Autodesk Inventor part; units mm, degrees
ref_plane "YZ Plane" through (0, 0, 0) normal (1, 0, 0) x (0, 1, 0)
ref_plane "XZ Plane" through (0, 0, 0) normal (0, 1, 0) x (-1, 0, 0)
ref_plane "XY Plane" through (0, 0, 0) normal (0, 0, 1) x (1, 0, 0)
sketch "Sketch1" plane through (0, 0, 0) normal (0, 0, 1) x (1, 0, 0)
  line L0 (145, 65) -> (-145, 65)
  line L1 (-145, 65) -> (-145, -65)
  line L2 (-145, -65) -> (145, -65)
  line L3 (145, -65) -> (145, 65)
  line L4 (145, 65) -> (-145, -65) construction
  line L5 (-145, 65) -> (145, -65) construction
  line L6 (85, 40) -> (-115, 40)
  line L7 (-115, 40) -> (-115, -40)
  line L8 (-115, -40) -> (85, -40)
  line L9 (85, -40) -> (85, 40)
  line L10 (85, 40) -> (-115, -40) construction
  line L11 (-115, 40) -> (85, -40) construction
  point P0 (0, 0)
  point P1 (0, 0)
  point P2 (-15, 0)
  point P3 (85, 0)
  point P4 (145, 0)
  dimension "d34" = 200
  dimension "d35" = 80
  dimension "d51" = 60
  dimension "d53" = 30
  dimension "d54" = 25
  dimension "d56" = 130
extrude "Plate1" add sketch "Sketch1" along normal blind 2
sketch "Sketch6" plane through (145, -63.5858, 1.4142) normal (0, -0.7071068, -0.7071068) x (1, 0, 0)
  line L0 (-290, 0) -> (0, 0)
  line L1 (0, 0) -> (0, 70)
  line L2 (0, 70) -> (-290, 70)
  line L3 (-290, 70) -> (-290, 0)
edge flange "Flange2" height 70 angle 45 thickness 2 bend radius 2.75 thickness toward (0, -0.7071068, -0.7071068) relief round relief width 2 relief depth 1 edges at (0, -65, 2) wall of the first edge with corners at (-145, -63.5858, 1.4142) (145, -63.5858, 1.4142) (145, -113.0833, 50.9117) (-145, -113.0833, 50.9117)
bend "Bend2"
corner "Corner2"
sketch "Sketch8" plane through (145, -112.4975, 49.4975) normal (0, -1, 0) x (1, 0, 0)
  line L0 (-290, 0) -> (0, 0)
  line L1 (0, 0) -> (0, 130)
  line L2 (0, 130) -> (-290, 130)
  line L3 (-290, 130) -> (-290, 0)
edge flange "Flange3" height 130 angle 45 thickness 2 bend radius 2.75 thickness toward (0, -1, 0) relief round relief width 2 relief depth 1 edges at (0, -113.0833, 50.9117) wall of the first edge with corners at (-145, -112.4975, 49.4975) (145, -112.4975, 49.4975) (145, -112.4975, 179.4975) (-145, -112.4975, 179.4975)
bend "Bend3"
corner "Corner3"
sketch "Sketch9" plane through (145, -113.0833, 178.0833) normal (0, -0.7071068, 0.7071068) x (1, 0, 0)
  line L0 (-290, 0) -> (0, 0)
  line L1 (0, 0) -> (0, 68.6)
  line L2 (0, 68.6) -> (-290, 68.6)
  line L3 (-290, 68.6) -> (-290, 0)
edge flange "Flange4" height 68.6 angle 45 thickness 2 bend radius 2.75 thickness toward (0, -0.7071068, 0.7071068) relief round relief width 2 relief depth 1 edges at (0, -112.4975, 179.4975) wall of the first edge with corners at (-145, -113.0833, 178.0833) (145, -113.0833, 178.0833) (145, -64.5757, 226.5908) (-145, -64.5757, 226.5908)
bend "Bend4"
corner "Corner4"
sketch "Sketch10" plane through (-145, -114.4975, 51.465) normal (0, -1, 0) x (1, 0, 0)
  line L0 (290, 126.065) -> (0, 126.065)
  line L1 (0, 0) -> (0, 126.065)
  line L2 (0, 0) -> (290, 0)
  line L3 (290, 126.065) -> (290, 0)
  line L4 (30, 23.0325) -> (230, 23.0325)
  line L5 (230, 23.0325) -> (230, 103.0325)
  line L6 (230, 103.0325) -> (30, 103.0325)
  line L7 (30, 103.0325) -> (30, 23.0325)
  point P0 (145, -51.465)
  point P1 (30, 63.0325)
  point P2 (0, 63.0325)
  dimension "d77" = 80
  dimension "d78" = 200
  dimension "d79" = 30
extrude "Cut3" cut sketch "Sketch10" against normal blind 2 contours L7 L6 L5 L4
equation "\"d34\" = MAIN_6_central_window_hight"
equation "\"d35\" = MAIN_7_central_window_width"
equation "\"d56\" = Wall_1_width"
equation "\"d77\" = MAIN_7_central_window_width"
equation "\"d78\" = MAIN_6_central_window_hight"
equation "\"d79\" = d53"
equation "\"d80\" = Thickness"
equation "\"d2\" = Thickness"
equation "\"d36\" = BendReliefWidth"
equation "\"d37\" = BendReliefDepth"
equation "\"d38\" = MinimumRemnant"
equation "\"d39\" = TransitionRadius"
equation "\"d40\" = Wall_2_width"
equation "\"d42\" = BendRadius"
equation "\"d43\" = CornerReliefSize"
equation "\"d44\" = GapSize"
equation "\"d45\" = JacobiRadiusSize"
equation "\"d57\" = BendReliefWidth"
equation "\"d58\" = BendReliefDepth"
equation "\"d59\" = MinimumRemnant"
equation "\"d60\" = TransitionRadius"
equation "\"d61\" = d56"
equation "\"d63\" = BendRadius"
equation "\"d64\" = CornerReliefSize"
equation "\"d65\" = GapSize"
equation "\"d66\" = JacobiRadiusSize"
equation "\"d67\" = BendReliefWidth"
equation "\"d68\" = BendReliefDepth"
equation "\"d69\" = MinimumRemnant"
equation "\"d70\" = TransitionRadius"
equation "\"d71\" = Wall_2_width - 0.7 * Thickness"
equation "\"d73\" = BendRadius"
equation "\"d74\" = CornerReliefSize"
equation "\"d75\" = GapSize"
equation "\"d76\" = JacobiRadiusSize"
equation "\"BendReliefWidth\" = Thickness"
equation "\"BendReliefDepth\" = 0.5 * Thickness"
equation "\"CornerReliefSize\" = 4 * Thickness"
equation "\"MinimumRemnant\" = 2 * Thickness"
equation "\"TransitionRadius\" = BendRadius"
equation "\"JacobiRadiusSize\" = BendRadius"
equation "\"GapSize\" = Thickness"
properties part number "TKS 3554 BOTTOM DS box wall 1" material "Stainless Steel"
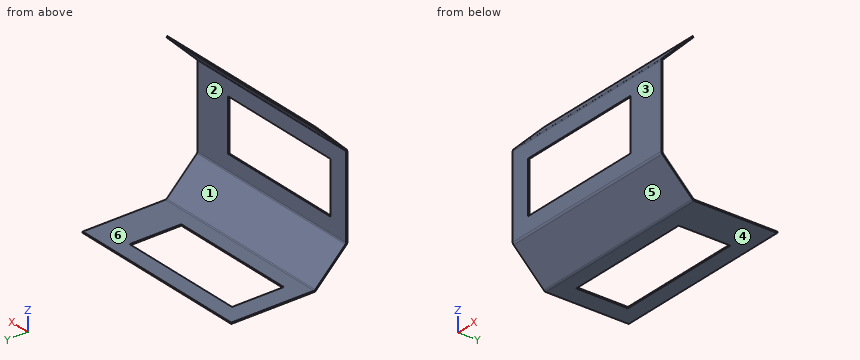
For this review, take the finished solid that the model builds, in its own axes (mm). Face numbers are marked on the shaded views. A direction names the side the tool comes from. Round coordinates to 2 decimals unless told otherwise and drop trailing zeros. Loops run counter-clockwise (first coordinate to the right, second up) from the corner with the lowest first, then second, coordinate; pieces in that order, holes last. Notation, with made-up numbers: (82, 44.5) - (114, 44.5) arc R19 ccw to (114, 58.5) - close; hole circle Ø1 at (9.5, -6). An arc over 180 degrees is marked (long way). One line per item, written item: value. Start each with the question number.
Item 1: Take a section at D-D (x = 105.5). Give the boundary of the cut face in (y, z), plus the area to 3 significant figures.
Item 2: For L1, parallel to Y at x = -117, z = 132; L2, parallel to Z at x = 56.5, y = -51; L3, parallel to Y at x = -116.5, z = 198.5, list the stretches that pass through material, from the lowest coordinate up.
Item 3: Take a section at B-B (z = 122.5). Give the boundary of the cut face in (x, y), plus the area to 3 significant figures.
Item 4: Take a section at A-A (y = -10.5). Give the boundary of the cut face in (x, z), plus the area to 3 significant figures.
Item 5: Clearance check with flat-ended pins moving along their axes: pin 1 Ø10 at (x, z) = (-36, 175) entering from +Y; pin 2 Ø1 at (x, y) = (-12.5, -113.5) entering from +Z (3 decimals); pin 3 Ø12 at (x, y) = (-104.5, 32.5) entering from -Z; pin 4 Ø1.5 at (x, z) = (92, 191) entering from +Y. State where each tip first meets the part, or that it passes through.
Item 6: For the marked faces 5 and 6, list the 3-axis set-ups (+Z, -Z, +X, -X, +Y, -Y) from which the entire face can be reached by the end or side of a thin tool; tool diameter is ignored.
Item 7: The part is to be moulded in two halves that separate along Z. For the marked faces 1, 2, 3 and 4, say which applies: +Z half, -Z half, draft (parallel to the pull), parting line (faces both ways), or undercut.
Item 8: Take a section at C-C (x = 72). Give the boundary of the cut face in (y, z).
Answer below:
1. outline: (-114.5, 51.46) arc R4.75 ccw to (-113.11, 48.11) - (-66.39, 1.39) arc R4.75 ccw to (-63.03, 0) - (65, 0) - (65, 2) - (-63.03, 2) arc R2.75 cw to (-64.98, 2.81) - (-111.69, 49.52) arc R2.75 cw to (-112.5, 51.46) - (-112.5, 177.53) arc R2.75 cw to (-111.69, 179.47) - (-64.58, 226.59) - (-65.99, 228.01) - (-113.11, 180.89) arc R4.75 ccw to (-114.5, 177.53) - close
1. area: 791 mm2
2. L1: y = -114.5 to -112.5
2. L2: z = 0 to 2
2. L3: y = -95.49 to -92.67
3. outline: (-145, -114.5) - (-115, -114.5) - (-115, -112.5) - (-145, -112.5) - close; (85, -114.5) - (145, -114.5) - (145, -112.5) - (85, -112.5) - close
3. area: 180 mm2
4. outline: (-145, 0) - (-115, 0) - (-115, 2) - (-145, 2) - close; (85, 0) - (145, 0) - (145, 2) - (85, 2) - close
4. area: 180 mm2
5. pin 1: stops at y = -111.17
5. pin 2: stops at z = 180.995
5. pin 3: passes through
5. pin 4: stops at y = -99.42
6. face 5: -Z, +X, -X, -Y
6. face 6: +Z, +X, -X, +Y
7. face 1: undercut
7. face 2: undercut
7. face 3: draft
7. face 4: -Z half
8. outline: (-114.5, 51.46) arc R4.75 ccw to (-113.11, 48.11) - (-66.39, 1.39) arc R4.75 ccw to (-63.03, 0) - (-40, 0) - (-40, 2) - (-63.03, 2) arc R2.75 cw to (-64.98, 2.81) - (-111.69, 49.52) arc R2.75 cw to (-112.5, 51.46) - (-112.5, 74.5) - (-114.5, 74.5) - close; (-114.5, 154.5) - (-112.5, 154.5) - (-112.5, 177.53) arc R2.75 cw to (-111.69, 179.47) - (-64.58, 226.59) - (-65.99, 228.01) - (-113.11, 180.89) arc R4.75 ccw to (-114.5, 177.53) - close; (40, 0) - (65, 0) - (65, 2) - (40, 2) - close
